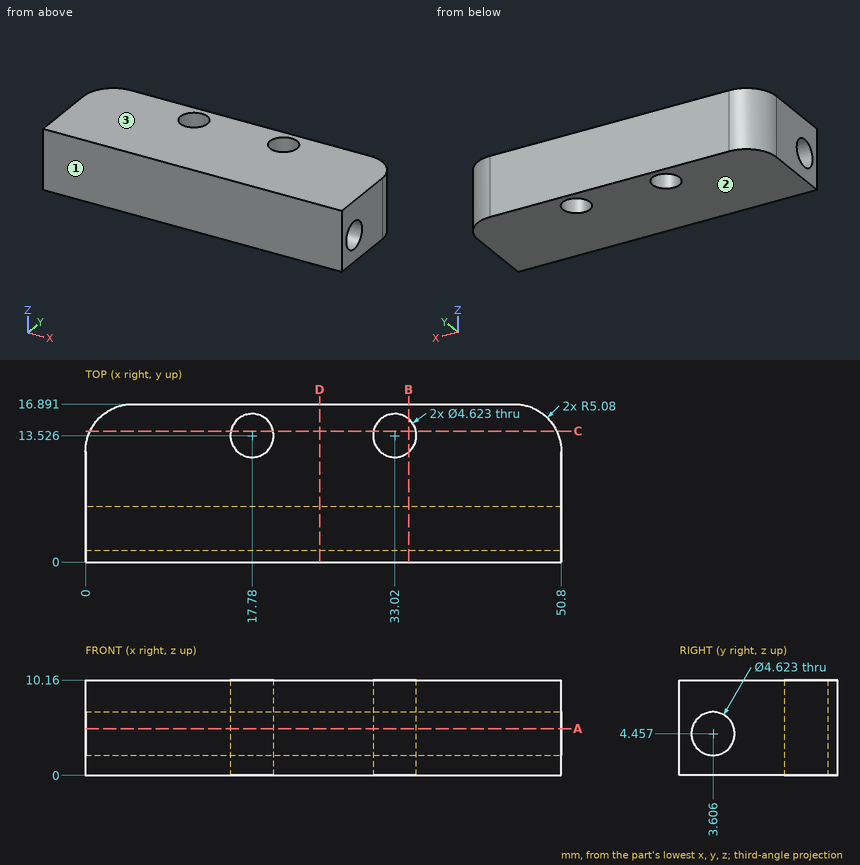
Input: dimensioned drawing with shaded views. Units: mm. Origin: part minimum x, y, z. Round coordinates to 2 decimals unless told otherwise and drop trailing zeros. Order: outer loops, then holes, each group sorted by start corner. A loop starts at its lowest first (then second) coordinate and runs counter-clockwise, first axis right, second up. Notation, with made-up numbers: (-36.75, -31) - (1.25, -31) arc R19 ccw to (1.25, 3) - close; hole circle Ø10 at (73.5, -5). An arc over 180 degrees is marked (long way). Write item = value, one per line. Start each with the question number.
Q1. Cut plane D-D on x = 25. Return the cut outline in (y, z) (1 decimal).
Q2. Cut plane B-B on x = 34.5. Give the number of separate pieces and of enclosed holes in the cut face, and give its area (3 significant figures).
Q3. Pin query (flat end, axial travel): pin 1 (5 mm diameter, centred on y = 15, z = 5, fed in from -X). Return the tip coordinate at first contact, or that it passes through.
Q4. Cut plane C-C on y = 14. Return the cut outline in (x, z) (1 decimal), and give its area (3 significant figures).
Q5. Ray query, line 1 (X direction, y = 14.75, z = 1) (1 decimal); line 2 (X direction, y = 14.5, z = 3.5) (1 decimal); line 3 (Y direction, x = 24, z = 5). Return the intervals inside material, ascending. Write a range as from..to.
Q6. Pull-direction query (Z, two-part tool) for the marked faces 1, 2 and 3; classes: +Z half, -Z half, draft (parallel to the pull), parting line (faces both ways), or undercut.
Q7. Cut plane A-A on z = 5. Return the cut outline in (x, y) (1 decimal), and give its area (3 significant figures).
Outcome:
q1.outline = (0, 0) - (16.9, 0) - (16.9, 10.2) - (0, 10.2) - close; hole circle Ø4.6 at (3.6, 4.5)
q2.separate_pieces = 2
q2.enclosed_holes = 1
q2.area = 119 mm^2
q3.pin_1 = 0.05
q4.outline = (0.5, 0) - (15.5, 0) - (15.5, 10.2) - (0.5, 10.2) - close; (20, 0) - (30.8, 0) - (30.8, 10.2) - (20, 10.2) - close; (35.3, 0) - (50.3, 0) - (50.3, 10.2) - (35.3, 10.2) - close
q4.area = 414 mm^2
q5.line_1 = 0.9..15.8, 19.7..31.1, 35..49.9
q5.line_2 = 0.8..15.7, 19.9..30.9, 35.1..50
q5.line_3 = 0..1.36, 5.85..16.89
q6.face_1 = draft
q6.face_2 = -Z half
q6.face_3 = +Z half
q7.outline = (0, 0) - (50.8, 0) - (50.8, 1.4) - (0, 1.4) - close; (0, 5.9) - (50.8, 5.9) - (50.8, 11.8) arc R5.1 ccw to (45.7, 16.9) - (5.1, 16.9) arc R5.1 ccw to (0, 11.8) - close; hole circle Ø4.6 at (17.8, 13.5); hole circle Ø4.6 at (33, 13.5)
q7.area = 585 mm^2
